The model under review builds one solid part; all positions refer to its coordinate system, in mm. Face numbers are marked on the shaded views. A direction names the side the tool comes from. Coordinates: 2 decimals unless noted, no trailing zeros. Loops run counter-clockwise (first coordinate to the right, second up) from the corner with the lowest first, then second, coordinate; pieces in that order, holes last. Notation, with made-up numbers: (54.5, -2.75) - (82.5, -2.75) arc R31 cw to (82.5, 22.25) - close; hole circle Ø2 at (-26.75, -9.5). An arc over 180 degrees is marked (long way). Use a Markdown table: item, result. Add a question column.
1) Add section C-C, the plane y = -23.75. Give the boundary of the cut face in (x, z), and give its area (3 significant figures).
2) Add section B-B, the plane y = -2.75. Give the boundary of the cut face in (x, z).
3) To check wall thickness, follow L1, parallel to X at y = -8, z = 19.5; L2, parallel to X at y = -4.5, z = 40.5; L3, parallel to Y at x = -13, z = 30.5. State the ranges of each line that lie inside material, in increasing order. Write a range as [from, to].
4) Add section A-A, the plane z = 23.5. Give the boundary of the cut face in (x, y).
5) Clearance check with a flat-ended pin moving along its axis: pin 1 (1.5 mm diameter, centred on x = -30.5, y = -8.5, fed in from +Z). State where the tip first meets the part, or that it passes through.
6) For the marked faces 1 and 2, list the 3-axis set-ups (+Z, -Z, +X, -X, +Y, -Y) from which the entire face can be reached by the end or side of a thin tool; tool diameter is ignored.
```python
from build123d import *

# Parameters (mm, degrees)
F1_DEPTH    = 25.4
F2_R        = 5.08
F3_T1_DEPTH = 27.7897108637
F3_T6_DEPTH = 5.1816


# Not quite as in the source:
# - a fillet or chamfer that OpenCascade refuses, or shapes differently, is made with other operations: its cross-section is extruded or revolved along the edge and cut away or added


with BuildPart() as f1:
    # F0 (on Front) → F1 (new body)
    with BuildSketch(Plane.XZ):
        Polygon((-8.6416769773, 61.5346953273), (-58.7037988007, 62.1306672692), (-58.7037988007, 17.1343572438), (-8.6416769773, 17.1343572438), align=None)
    extrude(amount=F1_DEPTH)

    # F2
    f2_edges = [f1.edges().sort_by_distance(p)[0] for p in [
        (-33.672738, -25.4, 61.832681),
        (-58.703799, -25.4, 39.632512),
        (-33.672738, -25.4, 17.134357),
        (-8.641677, -25.4, 39.334526),
        (-33.672738, 0, 61.832681),
        (-58.703799, 0, 39.632512),
        (-33.672738, 0, 17.134357),
        (-8.641677, 0, 39.334526),
        (-58.703799, -12.7, 17.134357),
        (-8.641677, -12.7, 17.134357),
    ]]
    fillet(f2_edges, radius=F2_R)

    # F3: fillet of radius 5.08 on 5 edges, made by hand

    # F3_s2 → F3_t1 (cut)
    with BuildSketch(Plane.XZ.offset(-7.4697108637)):
        with BuildLine():
            ThreePointArc((-13.6612056499, 61.5944510496), (-10.1082579355, 60.0854695805), (-8.6416769773, 56.5148109818))
            Line((-8.6416769773, 56.5148109818), (-8.6416769773, 61.5346953273))
            Line((-8.6416769773, 61.5346953273), (-13.6612056499, 61.5944510496))
        make_face()
    extrude(amount=F3_T1_DEPTH, mode=Mode.SUBTRACT)


with BuildPart() as f3_tool4:
    # F3_s5 → F3_t6 (new body)
    with BuildSketch(Plane.XZ.offset(20.32)):
        Polygon((-13.7216769773, 56.5148109818), (-13.6599962234, 61.696043851), (-8.5400769773, 61.6350930142), (-8.5400769773, 56.5148109818), align=None)
    extrude(amount=F3_T6_DEPTH)

    # F3_s7 → F3_t8 (revolve, cut)
    with BuildSketch(Plane(origin=(-13.7216769773, -20.32, 56.5148109818), x_dir=(-0.711302961, 0, -0.7028855509), z_dir=(-0.7028855509, 0, 0.711302961))):
        with BuildLine():
            ThreePointArc((0, -5.08), (5.08, 0), (0, 5.08))
            Line((0, 5.08), (0, -5.08))
        make_face()
    revolve(axis=Axis((-13.7216769773, -20.32, 56.5148109818), (0, -1, 0)), mode=Mode.SUBTRACT)


with BuildPart() as f1_1:
    add(f1.part)

    # F3_t3: cut F3_tool4
    add(f3_tool4.part, mode=Mode.SUBTRACT)


solid = f1_1.part
```
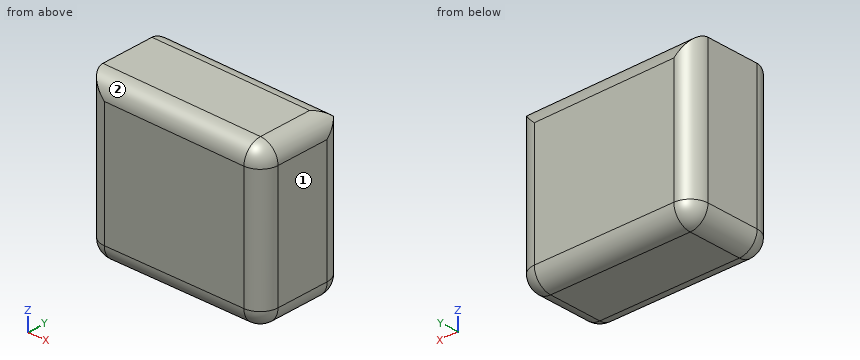
From the geometry:
| question | item | result |
|---|---|---|
| 1 | outline | (-57.37, 22.21) arc R3.75 ccw to (-53.62, 18.47) - (-13.72, 18.47) arc R3.75 ccw to (-9.97, 22.21) - (-9.97, 56.51) arc R3.75 ccw to (-13.68, 60.26) - (-57.37, 60.78) - close |
| 1 | area | 1,980 mm^2 |
| 2 | outline | (-58.14, 22.21) arc R4.51 ccw to (-53.62, 17.7) - (-13.72, 17.7) arc R4.51 ccw to (-9.21, 22.21) - (-9.21, 58.84) arc R5.08 ccw to (-11.34, 61) - (-58.14, 61.56) - close |
| 3 | L1 | x = [-57.92, -9.43] |
| 3 | L2 | x = [-58.67, -8.67] |
| 3 | L3 | y = [-25.35, -0.05] |
| 4 | outline | (-58.7, -20.32) arc R5.08 ccw to (-53.62, -25.4) - (-13.72, -25.4) arc R5.08 ccw to (-8.64, -20.32) - (-8.64, -5.08) arc R5.08 ccw to (-13.72, 0) - (-53.62, 0) arc R5.08 ccw to (-58.7, -5.08) - close |
| 5 | pin 1 | stops at z = 61.8 |
| 6 | face 1 | +Z, -Z, +X, +Y, -Y |
| 6 | face 2 | +Z, +X, -Y |
